Geometry: see drawing. Coordinates: mm, zero at the bounding-box minimum. A direction names the side the tool comes from. Round coordinates to 2 decimals unless told otherwise and drop trailing zeros. Loops run counter-clockwise (first coordinate to the right, second up) from the corner with the lowest first, then second, coordinate; pieces in that order, holes last.
(1) First-contact query: pin 1 Ø2 at (x, z) = (1.5, 5) entering from -Y; pin 2 Ø3.5 at (x, y) = (4.5, 22) entering from -Z; pin 3 Ø1.6 at (x, y) = (6.5, 9.5) entering from +Z. Flat tips, straight axial feed; report the tip coordinate or a pass-through.
(2) Set-up query: the marked faces 1, 2, 3, 4 and 5. Return all of +Z, -Z, +X, -X, +Y, -Y with unobstructed straight access to the full face (end or side cutting, diameter ignored); none if empty.
(3) Section A-A, the plane z = 25. Return the cut outline in (x, y).
(4) Section C-C, the plane y = 17. Return the cut outline in (x, z), plus the area to 3 significant figures.
(5) Material intervals for probe 1 along Y at (x, z) = (11.75, 10); probe 2 along Z at (x, y) = (3.5, 9.25), sorted ascending.
(6) Section D-D, the plane z = 3. Return the cut outline in (x, y), plus the area to 3 significant figures.
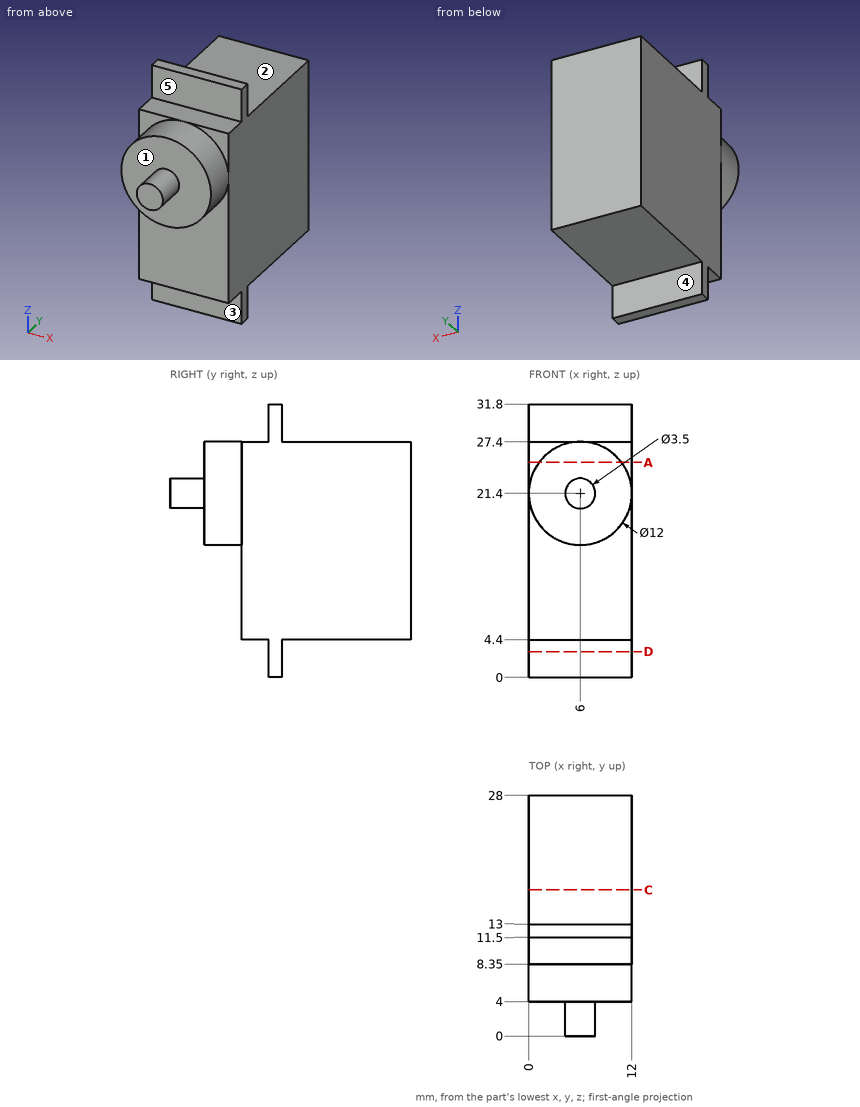
Output values:
1. pin 1: stops at y = 8.35
1. pin 2: stops at z = 4.4
1. pin 3: stops at z = 27.4
2. face 1: -Y
2. face 2: +Z, +X, -X, +Y
2. face 3: -Z, +X, -X, -Y
2. face 4: -Z, +X, -X, +Y
2. face 5: +Z, +X, -X, -Y
3. outline: (0, 8.35) - (1.2, 8.35) - (1.2, 4) - (10.8, 4) - (10.8, 8.35) - (12, 8.35) - (12, 28) - (0, 28) - close
4. outline: (0, 4.4) - (12, 4.4) - (12, 27.4) - (0, 27.4) - close
4. area: 276 mm2
5. probe 1: y = 8.35 to 28
5. probe 2: z = 4.4 to 27.4
6. outline: (0, 11.5) - (12, 11.5) - (12, 13) - (0, 13) - close
6. area: 18.0 mm2
